For this review, take the finished solid that the model builds, in its own axes (mm). Coordinates: 2 decimals unless noted, no trailing zeros. Loops run counter-clockwise (first coordinate to the right, second up) from the corner with the lowest first, then second, coordinate; pieces in that order, holes last. Notation, with made-up numbers: M 34,50.25 L 38,50.25 A27 cw 38,77.25 Z; hole C 74.5,-1.5 d11. An arc over 180 degrees is marked long. Write item = value, one per line.
from build123d import *

# Parameters (mm, degrees)
SKETCH1_W           = 152
SKETCH1_H           = 120
SKETCH1_R           = 2.5
SKETCH1_R_2         = 11
BOSS_EXTRUDE1_DEPTH = 3
SKETCH2_R           = 2
CUT_EXTRUDE1_DEPTH  = 4


with BuildPart() as part:
    # Sketch1 → Boss-Extrude1 (new body)
    with BuildSketch(Plane(origin=(0, 0, 0), x_dir=(1, 0, 0), z_dir=(0, 1, 0))):
        with Locations((49.311456102, 37.795094937)):
            Rectangle(SKETCH1_W, SKETCH1_H)
        with Locations((24.311456102, 17.795094937)):
            Circle(SKETCH1_R, mode=Mode.SUBTRACT)
        with Locations((34.311456102, 17.795094937)):
            Circle(SKETCH1_R, mode=Mode.SUBTRACT)
        with Locations((64.311456102, 17.795094937)):
            Circle(SKETCH1_R, mode=Mode.SUBTRACT)
        with Locations((74.311456102, 17.795094937)):
            Circle(SKETCH1_R, mode=Mode.SUBTRACT)
        with Locations((29.311456102, 37.795094937)):
            Circle(SKETCH1_R_2, mode=Mode.SUBTRACT)
        with Locations((69.311456102, 37.795094937)):
            Circle(SKETCH1_R_2, mode=Mode.SUBTRACT)
    extrude(amount=BOSS_EXTRUDE1_DEPTH)

    # Sketch2 → Cut-Extrude1 (cut, through all)
    with BuildSketch(Plane.XZ):
        with Locations((4.327840203, 2.482417514)):
            Circle(SKETCH2_R)
        with Locations((95.311456102, -79.795094937)):
            Circle(SKETCH2_R)
        with Locations((3.311456102, -79.795094937)):
            Circle(SKETCH2_R)
        with Locations((-8.688543898, -82.997135966)):
            Circle(SKETCH2_R)
        with Locations((95.311456102, 4.204905063)):
            Circle(SKETCH2_R)
        with Locations((107.311456102, -82.997135966)):
            Circle(SKETCH2_R)
        with Locations((-8.688543898, 7.406946092)):
            Circle(SKETCH2_R)
        with Locations((107.311456102, 7.406946092)):
            Circle(SKETCH2_R)
    extrude(amount=-CUT_EXTRUDE1_DEPTH, mode=Mode.SUBTRACT)


solid = part.part
Q1. Draft analysis for pull direction X (two halves, no side actions). For faces 1 (the face through (-26.689, 1, -37)), 2 (the face through (48, 1, 22.205)), 3 (the face through (66.696, 1.479, -18.546)), state which applies: +X half, -X half, draft (parallel to the pull), parting line (faces both ways), or undercut.
Solved:
face_1 = -X half
face_2 = draft
face_3 = undercut
Q2. Add section C-C (x = 95.5). Write out the cut boundary in (y, z).
Solved:
outline = M 0,-97.8 L 3,-97.8 L 3,-81.79 L 0,-81.79 Z; M 0,-77.8 L 3,-77.8 L 3,2.21 L 0,2.21 Z; M 0,6.2 L 3,6.2 L 3,22.2 L 0,22.2 Z
Q3. Add section A-A (x = 63.5). Write out the cut boundary in (y, z), and give its area (3 significant figures).
Solved:
outline = M 0,-97.8 L 3,-97.8 L 3,-47.13 L 0,-47.13 Z; M 0,-28.46 L 3,-28.46 L 3,-20.16 L 0,-20.16 Z; M 0,-15.43 L 3,-15.43 L 3,22.2 L 0,22.2 Z
area = 290 mm²
Q4. Add section B-B (y = 1.7). State how many separate pieces and enclosed holes the cut face has, and give its area (3 significant figures).
Solved:
separate_pieces = 1
enclosed_holes = 14
area = 17,300 mm²
Q5. For line 1 along Z through (x, y) = (75.5, 2.55); line 2 along X through (y, z) = (2.95, -46); line 3 along X through (y, z) = (0.4, -16), list the stretches that pass through material, from the lowest coordinate up.
Solved:
line_1 = -97.8 to -46.89, -28.7 to -19.99, -15.6 to 22.2
line_2 = -26.69 to 21.98, 36.64 to 61.98, 76.64 to 125.31
line_3 = -26.69 to 22.57, 26.05 to 32.57, 36.05 to 62.57, 66.05 to 72.57, 76.05 to 125.31
Q6. For pin 1 Ø6.5 at (x, z) = (95.31, -79.8) entering from +Y, flat-tipped, find the tip position at first contact; note if it passes through.
Solved:
pin_1 = 3
